from build123d import *

# Parameters (mm, degrees)
F0_W     = 57.15
F0_H     = 44.45
F1_DEPTH = 25.4
F3_DEPTH = 12.7
F5_DEPTH = 25.4


with BuildPart() as f1:
    # F0 (on Front) → F1 (new body)
    with BuildSketch(Plane.XZ):
        with Locations((28.575, 22.225)):
            Rectangle(F0_W, F0_H)
    extrude(amount=F1_DEPTH)

    # F2 (on face) → F3 (cut)
    with BuildSketch(Plane.XZ.offset(25.4)):
        Polygon((19.05, 44.45), (44.45, 0), (57.15, 0), (57.15, 44.45), align=None)
    extrude(amount=-F3_DEPTH, mode=Mode.SUBTRACT)

    # F4 (on face) → F5 (cut)
    with BuildSketch(Plane.XZ.offset(25.4)):
        with BuildLine():
            ThreePointArc((35.143775, 16.285894), (38.674012, 19.792631), (39.967225, 24.597564))
            ThreePointArc((39.967225, 24.597564), (35.199182, 32.877327), (25.644724, 32.909234))
            Line((25.644724, 32.909234), (35.143775, 16.285894))
        make_face()
        with BuildLine():
            Line((35.143775, 16.285894), (25.644724, 32.909234))
            ThreePointArc((25.644724, 32.909234), (22.082579, 19.848038), (35.143775, 16.285894))
        make_face()
    extrude(amount=-F5_DEPTH, mode=Mode.SUBTRACT)


solid = f1.part
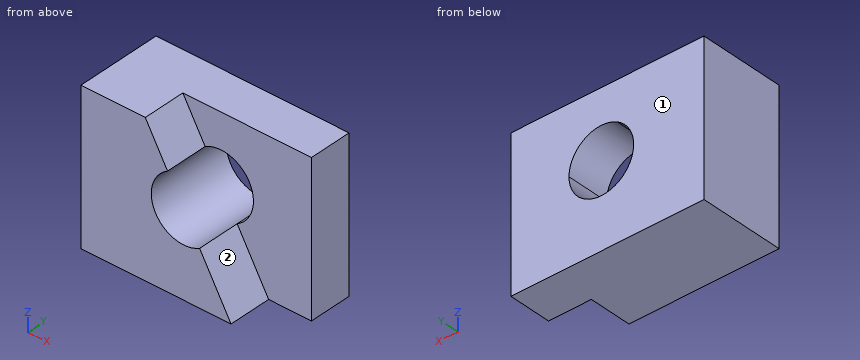
Input: part model. Units: mm. Frame: model coordinates. Face numbers are marked on the shaded views. A direction names the side the tool comes from. Give positions to 0.01 mm unless a question says otherwise; leave off trailing zeros. Order: outer loops, then holes, each group sorted by start corner. A loop starts at its lowest first (then second) coordinate and runs counter-clockwise, first axis right, second up.
Q1. Section C-C on y = -6.75. Output: boundary loops of the cut face in (x, z).
Checked values:
outline: (0, 0) - (57.15, 0) - (57.15, 44.45) - (0, 44.45) - close; hole (35.14, 16.29) arc R9.57 ccw to (39.97, 24.6) arc R9.57 ccw (long way) to start
Q2. Contact query for flat-ended pins moving along their axis: pin 1 Ø1.5 at (x, z) = (41, 17) entering from -Y; pin 2 Ø2 at (x, y) = (41.5, -21.5) entering from +Z. Output: stop coordinate, or through.
Checked values:
pin 1: stops at y = -12.7
pin 2: stops at z = 6.91
Q3. Ray query, probe 1 along X at (y, z) = (-15, 24.5); probe 2 along Y at (x, z) = (43.5, 30); probe 3 along X at (y, z) = (-8.25, 29). Return the intervals inside material, ascending.
Checked values:
probe 1: x = 0 to 20.82
probe 2: y = -12.7 to 0
probe 3: x = 0 to 21.89, 38.89 to 57.15
Q4. Section B-B on z = 17.5. Output: boundary loops of the cut face in (x, y), and give its area (3 significant figures).
Checked values:
outline: (0, -25.4) - (23.97, -25.4) - (23.97, 0) - (0, 0) - close; (36.82, -12.7) - (57.15, -12.7) - (57.15, 0) - (36.82, 0) - close
area: 867 mm2
Q5. Set-up query: the marked faces 1 and 2. Return all of +Z, -Z, +X, -X, +Y, -Y with unobstructed straight access to the full face (end or side cutting, diameter ignored); none if empty.
Checked values:
face 1: +Z, -Z, +X, -X, +Y
face 2: +Z, +X, -Y
Q6. Section D-D on y = -19. Output: boundary loops of the cut face in (x, z), and give its area (3 significant figures).
Checked values:
outline: (0, 0) - (44.45, 0) - (35.14, 16.29) arc R9.57 cw to (25.64, 32.91) - (19.05, 44.45) - (0, 44.45) - close
area: 1,270 mm2
Q7. Section A-A on x = 22. Output: boundary loops of the cut face in (y, z).
Checked values:
outline: (-25.4, 0) - (0, 0) - (0, 20) - (-25.4, 20) - close; (-25.4, 29.2) - (0, 29.2) - (0, 44.45) - (-12.7, 44.45) - (-12.7, 39.29) - (-25.4, 39.29) - close
